Design review of the part built by this model. Coordinates are the model's own, in mm. Coordinates: 2 decimals unless noted, no trailing zeros. Loops run counter-clockwise (first coordinate to the right, second up) from the corner with the lowest first, then second, coordinate; pieces in that order, holes last. Notation, with made-up numbers: M -37.5,-14 L 16.5,-14 A37 ccw 16.5,23 Z; hole C 58,77.25 d3. An arc over 180 degrees is marked long. One line per item, written item: value.
```python
from build123d import *

# Parameters (mm, degrees)
SKETCH5_W           = 42
SKETCH5_H           = 23
BOSS_EXTRUDE2_DEPTH = 32
CUT_EXTRUDE3_DEPTH  = 42


with BuildPart() as part:
    # Sketch5 → Boss-Extrude2 (new body)
    with BuildSketch(Plane.XY.offset(-10)):
        Rectangle(SKETCH5_W, SKETCH5_H)
    extrude(amount=-BOSS_EXTRUDE2_DEPTH)

    # Sketch6 → Cut-Extrude3 (cut)
    with BuildSketch(Plane.ZY.offset(21)):
        Polygon((-42, 11.5), (-42, -8.5), (-15, 11.5), align=None)
    extrude(amount=-CUT_EXTRUDE3_DEPTH, mode=Mode.SUBTRACT)


solid = part.part
```
(1) Insertion check: pin 1 (1 mm diameter, centred on x = 1, z = -26.5, fed in from +Y). The pin has a flat end and moves straight along its axis. Give the tip position at first contact, or say it passes through.
Reply:
pin 1: stops at y = 3.35
(2) We need section A-A on x = 8. State the section outline as (y, z) points, then the cut area to 3 significant figures.
Reply:
outline: M -11.5,-42 L -8.5,-42 L 11.5,-15 L 11.5,-10 L -11.5,-10 Z
area: 466 mm2
(3) We need section B-B on y = -1.5. State the section outline as (x, z) points.
Reply:
outline: M -21,-32.55 L 21,-32.55 L 21,-10 L -21,-10 Z
(4) We need section C-C on z = -16. State the section outline as (x, y) points.
Reply:
outline: M -21,-11.5 L 21,-11.5 L 21,10.76 L -21,10.76 Z
(5) To check wall thickness, follow line 1 along Z through (x, y) = (-8.5, 1.5); line 2 along Y through (x, z) = (-15.5, -39.5); line 3 along Z through (x, y) = (-14, -0.5). State the ranges of each line that lie inside material, in increasing order. Write a range as [from, to].
Reply:
line 1: z = [-28.5, -10]
line 2: y = [-11.5, -6.65]
line 3: z = [-31.2, -10]
